from build123d import *

# Parameters (mm, degrees)
F0_W     = 8.1
F0_H     = 18
F1_DEPTH = 1.8
F0_W_2   = 1.2
F0_W_3   = 2
F2_DEPTH = 8


# Not quite as in the source:
# - a feature names something its author has since deleted; it is built from what else it names


with BuildPart() as f1:
    # F0 (on Top) → F1 (new body)
    with BuildSketch(Plane.XY):
        Polygon((6.05, -9), (4.05, -9), (-4.05, -9), (-5.25, -9), (-5.25, -19), (6.05, -19), align=None)
        Rectangle(F0_W, F0_H)
        Polygon((6.05, 9), (6.05, -9), (6.05, -19), (12.05, -19), (12.05, 9), align=None)
    extrude(amount=F1_DEPTH)

    # F0 (on Top) → F2 (join)
    with BuildSketch(Plane.XY):
        with Locations((-4.65, 0)):
            Rectangle(F0_W_2, F0_H)
        with Locations((5.05, 0)):
            Rectangle(F0_W_3, F0_H)
    extrude(amount=F2_DEPTH)


solid = f1.part
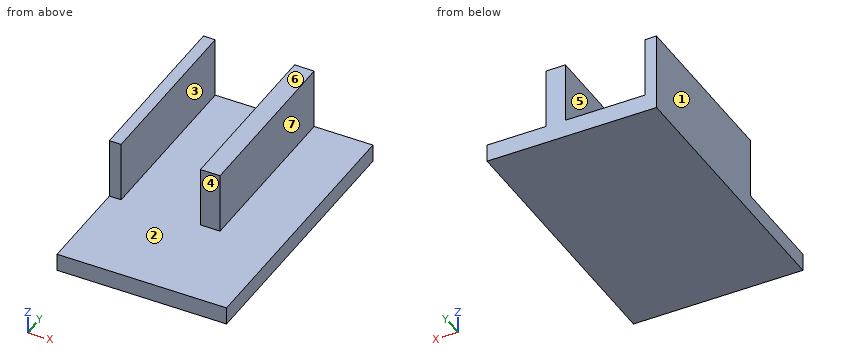
Read the model definition and answer for the solid it produces. Units are mm, in the model's axes. Face numbers are marked on the shaded views. A direction names the side the tool comes from. Coordinates: 2 decimals unless noted, no trailing zeros. Order: outer loops, then holes, each group sorted by start corner. A loop starts at its lowest first (then second) coordinate and runs counter-clockwise, first axis right, second up. Notation, with made-up numbers: (66, -36.5) -> (102, -36.5) arc R26 cw to (102, -19.5) -> close; hole circle Ø5 at (-5.5, 51). An arc over 180 degrees is marked (long way). Answer as a JSON object with one key per item and string values.
1) A cutting plane is placed at C-C, the plane x = 3. Determine the outline of the cut face in (y, z), plus the area to 3 significant figures.
Model answer:
{"outline": "(-19, 0) -> (9, 0) -> (9, 1.8) -> (-19, 1.8) -> close", "area": "50.4 mm²"}
2) A cutting plane is placed at D-D, the plane y = -14. Determine the outline of the cut face in (x, z), plus the area to 3 significant figures.
Model answer:
{"outline": "(-5.25, 0) -> (12.05, 0) -> (12.05, 1.8) -> (-5.25, 1.8) -> close", "area": "31.1 mm²"}
3) A cutting plane is placed at B-B, the plane y = 2.75. Determine the outline of the cut face in (x, z).
Model answer:
{"outline": "(-5.25, 0) -> (12.05, 0) -> (12.05, 1.8) -> (6.05, 1.8) -> (6.05, 8) -> (4.05, 8) -> (4.05, 1.8) -> (-4.05, 1.8) -> (-4.05, 8) -> (-5.25, 8) -> close"}
4) Consider line 1 along X through (y, z) = (3.5, 3.5); line 2 along Z through (x, y) = (2, -6.75). Determine where each line is inside the solid, lowest interval first. Write a range as from..to.
Model answer:
{"line 1": "x = -5.25..-4.05, 4.05..6.05", "line 2": "z = 0..1.8"}
5) The mould has two halves that part along X. Classify the marked faces 1, 2, 3 and 4: released by +X, released by -X, zero draft, split by the parting line, or undercut.
Model answer:
{"face 1": "released by -X", "face 2": "undercut", "face 3": "undercut", "face 4": "zero draft"}
6) Each of these flat-tipped pins is pushed along its axis until it touches: pin 1 (5 mm diameter, centred on x = 3.5, y = -11.5, fed in from +Z); pin 2 (1.9 mm diameter, centred on y = 2, z = 4, fed in from +X); pin 3 (0.6 mm diameter, centred on x = -4.5, z = 4.5, fed in from -Y). Where does it stop, or does it pass through?
Model answer:
{"pin 1": "stops at z = 1.8", "pin 2": "stops at x = 6.05", "pin 3": "stops at y = -9"}
7) A tool of negligible diameter and unlimited length cuts with its end or side. For the marked faces 5, 6 and 7, from which of +Z, -Z, +X, -X, +Y, -Y can it reach the whole face along a straight path? Write none if from no direction.
Model answer:
{"face 5": "+Z, +Y, -Y", "face 6": "+Z, +X, -X, +Y, -Y", "face 7": "+Z, +X, +Y, -Y"}
8) A cutting plane is placed at A-A, the plane z = 6.25. Determine the outline of the cut face in (x, y).
Model answer:
{"outline": "(-5.25, -9) -> (-4.05, -9) -> (-4.05, 9) -> (-5.25, 9) -> close; (4.05, -9) -> (6.05, -9) -> (6.05, 9) -> (4.05, 9) -> close"}
